Model file for the job. Use its own axes, mm. Face numbers are marked on the shaded views. A direction names the side the tool comes from. Give positions to 0.01 mm unless a question says otherwise; leave off trailing zeros. Loops run counter-clockwise (first coordinate to the right, second up) from the corner with the lowest first, then second, coordinate; pieces in that order, holes last. Notation, with made-up numbers: M 54,5.5 L 109,5.5 A6 ccw 109,13.5 Z; hole C 88,-7.5 d9. An arc over 180 degrees is marked long. Answer in a Markdown table with one row per item.
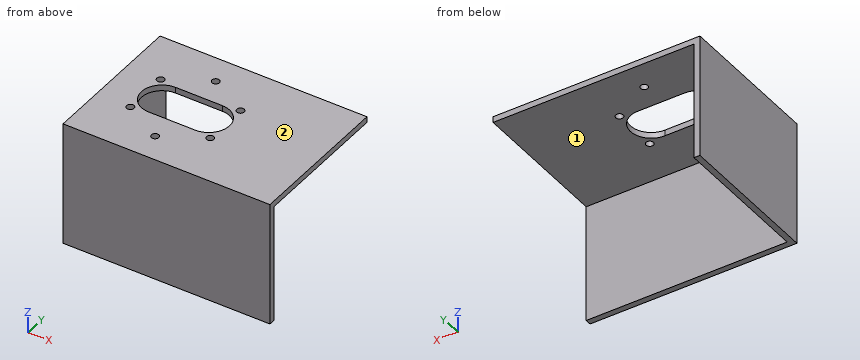
Autodesk Inventor part; units mm, degrees
ref_plane "YZ Plane" through (0, 0, 0) normal (1, 0, 0) x (0, 1, 0)
ref_plane "XZ Plane" through (0, 0, 0) normal (0, 1, 0) x (-1, 0, 0)
ref_plane "XY Plane" through (0, 0, 0) normal (0, 0, 1) x (1, 0, 0)
sketch "Sketch1" plane through (0, 0, 0) normal (0, 0, 1) x (1, 0, 0)
  circle A0 centre (0, 0) radius 18.38
  circle A1 centre (13.5143, 7.8025) radius 1.255
  circle A2 centre (0, 15.605) radius 1.255
  circle A3 centre (-13.5143, 7.8025) radius 1.255
  circle A4 centre (-13.5143, -7.8025) radius 1.255
  circle A5 centre (0, -15.605) radius 1.255
  circle A6 centre (13.5143, -7.8025) radius 1.255
  circle A7 centre (7.9, 0) radius 5.98
  line L0 (25, 25) -> (-25, 25)
  line L1 (-25, 25) -> (-25, -25)
  line L2 (-25, -25) -> (25, -25)
  line L3 (25, -25) -> (25, 25)
  line L4 (25, 25) -> (-25, -25) construction
  line L5 (-25, 25) -> (25, -25) construction
  circle A8 centre (7.9, 0) radius 6.98
  line L6 (7.9, -6.98) -> (-7.9, -6.98)
  line L7 (7.9, 6.98) -> (-7.9, 6.98)
  circle A9 centre (-7.9, 0) radius 6.98
  line L8 (23, 23) -> (-23, 23)
  line L9 (-23, 23) -> (-23, -23)
  line L10 (-23, -23) -> (23, -23)
  line L11 (23, -23) -> (23, 23)
  line L12 (-23, 23) -> (-23, 25)
  line L13 (23, 23) -> (23, 25)
  line L14 (23, -23) -> (23, -25)
  line L15 (23, -23) -> (25, -23)
  point P0 (0, 0)
  dimension "d0" = 50
  dimension "d1" = 50
  dimension "d2" = 1
  dimension "d3" = 15.8
  dimension "d6" = 2
extrude "Extrusion1" add sketch "Sketch1" along normal blind 2 contours A0 | L3 L15 L11 L13 L0 | L13 L8 L12 L0 | L3 L2 L14 L15 | L12 L9 L10 L14 L2 L1 L0 | L11 L10 L9 L8
extrude "Extrusion2" add sketch "Sketch1" against normal blind 40 contours L3 L2 L14 L15 | L12 L9 L10 L14 L2 L1 L0
thread "Thread1"
thread "Thread2"
thread "Thread3"
thread "Thread4"
thread "Thread5"
thread "Thread6"
sketch "Sketch2" plane through (25, -25, 0) normal (1, 0, 0) x (0, 0, -1)
  line L0 (0, 2) -> (0, 50)
  line L1 (0, 2) -> (40, 2)
  line L2 (40, 2) -> (40, 0)
  line L3 (0, 0) -> (40, 0)
  line L4 (40, 0) -> (-2, 0)
  line L5 (-2, 0) -> (-2, 50)
  line L6 (0, 50) -> (-2, 50)
  point P0 (0, 25)
extrude "Extrusion3" add sketch "Sketch2" along normal blind 20
properties part number "extendeddrivemotorcasing"
Q1. Saw through at C-C (z = -32). Give the cut face in (x, y), and give its area (3 significant figures).
Reported:
| item | result |
|---|---|
| outline | M -25,-25 L 45,-25 L 45,-23 L -23,-23 L -23,25 L -25,25 Z |
| area | 236 mm² |
Q2. 3-axis set-ups, long thin cutter, end or side, ignore diameter. For the marked faces 1 and 2: which of +Z, -Z, +X, -X, +Y, -Y reach the whole face in a straight line?
Reported:
| item | result |
|---|---|
| face 1 | -Z, +X, +Y |
| face 2 | +Z, +X, -X, +Y, -Y |
Q3. Saw through at D-D (x = 27). Give the cut face in (y, z), and give its area (3 significant figures).
Reported:
| item | result |
|---|---|
| outline | M -25,-40 L -23,-40 L -23,0 L 25,0 L 25,2 L -25,2 Z |
| area | 180 mm² |
Q4. Drop flat-ended pins along their axis: pin 1 (12 mm diameter, centred on x = -12.5, z = -17, fed in from +Y); pin 2 (8 mm diameter, centred on y = -3, z = -26, fed in from +X); pin 3 (10 mm diameter, centred on x = 37, y = -17.5, fed in from -Z). Give the stop position or say it passes through.
Reported:
| item | result |
|---|---|
| pin 1 | y = -23 |
| pin 2 | x = -23 |
| pin 3 | z = 0 |
Q5. Saw through at A-A (y = 0). Give the cut face in (x, z), and give its area (3 significant figures).
Reported:
| item | result |
|---|---|
| outline | M -25,-40 L -23,-40 L -23,0 L -14.88,0 L -14.88,2 L -25,2 Z; M 14.88,0 L 45,0 L 45,2 L 14.88,2 Z |
| area | 160 mm² |
Q6. Probe probe 1 along Y at (x, z) = (0, 1); probe 2 along Z at (x, y) = (19.5, -6.5); probe 3 along Y at (x, z) = (-13.5, -9). List the from-to ranges inside material, lowest first.
Reported:
| item | result |
|---|---|
| probe 1 | -25 to -16.86, -14.35 to -6.98, 6.98 to 14.35, 16.86 to 25 |
| probe 2 | 0 to 2 |
| probe 3 | -25 to -23 |
Q7. Saw through at B-B (x = -6). Give the cut face in (y, z), and give its area (3 significant figures).
Reported:
| item | result |
|---|---|
| outline | M -25,-40 L -23,-40 L -23,0 L -6.98,0 L -6.98,2 L -25,2 Z; M 6.98,0 L 25,0 L 25,2 L 6.98,2 Z |
| area | 152 mm² |
